Read the model definition and answer for the solid it produces. Units are mm, in the model's axes. Give positions to 0.01 mm unless a question says otherwise; leave off trailing zeros. Loops run counter-clockwise (first coordinate to the right, second up) from the corner with the lowest first, then second, coordinate; pieces in that order, holes last. Notation, with made-up numbers: M 11,-13 L 32,-13 A25 cw 32,6 Z; hole C 63,70.5 d3. An arc over 180 degrees is marked long. Return JSON: item names as keys, results as strings. Group by question number.
```python
from build123d import *

# Parameters (mm, degrees)
SKETCH_1_R      = 2.5
EXTRUDE_1_DEPTH = 5
EXTRUDE_2_DEPTH = 3


with BuildPart() as part:
    # 草图1 → 凸台-拉伸1 (new body)
    with BuildSketch(Plane.XY):
        Circle(SKETCH_1_R)
    extrude(amount=EXTRUDE_1_DEPTH)

    # 草图2 → 凸台-拉伸2 (add)
    with BuildSketch(Plane.XY.offset(5)):
        with BuildLine():
            Line((-0.184041749, 2.994349451), (-0.374222232, 2.471832867))
            ThreePointArc((-0.374222232, 2.471832867), (0, 2.5), (0.374222232, 2.471832867))
            Line((0.374222232, 2.471832867), (0.184041749, 2.994349451))
            ThreePointArc((0.184041749, 2.994349451), (0, 3), (-0.184041749, 2.994349451))
        make_face()
    extrude(amount=-EXTRUDE_2_DEPTH)


solid = part.part
```
1. Straight lines are drawn through the part: line 1 along X through (y, z) = (0.1, 1.15); line 2 along Y through (x, z) = (2.3, 4.4); line 3 along Y through (x, z) = (-2.1, 3.05). For each, find the intervals that lie inside material, in ascending order.
2. Find section B-B (z = 3.4). Write down the section's boundary in (x, y), and give its area (3 significant figures).
3. Find section D-D (z = 1.9). Write down the section's boundary in (x, y).
4. Find section C-C (y = -0.6). Write down the section's boundary in (x, z).
5. Flat-ended cylindrical pins translate along their axes: P1, Ø0.6, axis at x = 0, y = 3, coming from the -Z side; P2, Ø1.5, axis at y = -2, z = 2, coming from the +X side. Find the tip coordinate at first contact, or state that the pin passes through.
6. Find section A-A (x = 0). Write down the section's boundary in (y, z).
Result:
{
 "1": {"line 1": "x = -2.5 to 2.5", "line 2": "y = -0.98 to 0.98", "line 3": "y = -1.36 to 1.36"},
 "2": {"outline": "M -0.37,2.47 A2.5 ccw long 0.37,2.47 L 0.18,2.99 A3 ccw -0.18,2.99 Z", "area": "19.9 mm2"},
 "3": {"outline": "C 0,0 d5"},
 "4": {"outline": "M -2.43,0 L 2.43,0 L 2.43,5 L -2.43,5 Z"},
 "5": {"P1": "stops at z = 2", "P2": "stops at x = 2.17"},
 "6": {"outline": "M -2.5,0 L 2.5,0 L 2.5,2 L 3,2 L 3,5 L -2.5,5 Z"}
}
